from build123d import *

# Parameters (mm, degrees)
F0_R     = 15.24
F0_R_2   = 13.335
F0_R_3   = 8.89
F0_R_4   = 8.382
F1_DEPTH = 5.08
F2_DEPTH = 17.78
F3_DEPTH = 17.78


with BuildPart() as f1:
    # F0 (on Top) → F1 (new body)
    with BuildSketch(Plane.XY):
        Circle(F0_R)
        Circle(F0_R_2, mode=Mode.SUBTRACT)
        Circle(F0_R_2)
        Circle(F0_R_3, mode=Mode.SUBTRACT)
        Circle(F0_R_3)
        Circle(F0_R_4, mode=Mode.SUBTRACT)
        Circle(F0_R_4)
    extrude(amount=F1_DEPTH)

    # F0 (on Top) → F2 (join)
    with BuildSketch(Plane.XY):
        Circle(F0_R)
        Circle(F0_R_2, mode=Mode.SUBTRACT)
    extrude(amount=F2_DEPTH)

    # F0 (on Top) → F3 (join)
    with BuildSketch(Plane.XY):
        Circle(F0_R_3)
        Circle(F0_R_4, mode=Mode.SUBTRACT)
    extrude(amount=F3_DEPTH)


solid = f1.part
Here's how the part is built. I have some questions about the finished solid (model axes, mm). A direction names the side the tool comes from. Round coordinates to 2 decimals unless told otherwise and drop trailing zeros. Write each loop counter-clockwise with the first axis right and the second up, starting at its lowest first coordinate (ties: lowest second). Pieces come first, ordered by that corner, then holes.
1. If we mould it in two halves opening along Y, with no side actions, what happens to faces 3 (the cylindrical face through (-1.93, -8.68, 11.34)), 4 (the flat face through (-3, 8, 17.78)), 5 (the cylindrical face through (-3.3, -14.88, 8.77))? For each: released by +Y, released by -Y, zero draft, split by the parting line, or undercut.
2. Suppose I cut it at A-A (y = 0). List the corners of the cut face in (x, z) for me (3 decimals).
3. For faces 1 (the flat face through (0, 0, 0)), 2 (the cylindrical face through (-1.74, 13.22, 11.34)), which set-ups out of +Z, -Z, +X, -X, +Y, -Y let a thin tool reach every point of the face, with its end or its side?
4. I need wall thicknesses on L1, parallel to Y at x = 0, z = 10.75 (3 decimals); L2, parallel to Y at x = 4.5, z = 10.5; L3, parallel to Z at x = 6.5, y = 0. Which ranges of each line are inside material? Lowest first, please.
5. Suppose I cut it at D-D (z = 2.5). List the corners of the cut face in (x, y) for me, and give its area (3 significant figures).
6. Will these pins go through, and if not, where does the flat tip stop? pin 1 Ø1.5 at (y, z) = (3.5, 12.5) entering from -X; pin 2 Ø5 at (x, y) = (-3, 0) entering from +Z; pin 3 Ø4 at (x, z) = (-9.5, 11) entering from +Y.
7. Suppose I cut it at B-B (z = 9). List the corners of the cut face in (x, y) for me (3 decimals), and give its area (3 significant figures).
Answer sheet:
1. face 3: undercut
1. face 4: zero draft
1. face 5: split by the parting line
2. outline: (-15.24, 0) - (15.24, 0) - (15.24, 17.78) - (13.335, 17.78) - (13.335, 5.08) - (8.89, 5.08) - (8.89, 17.78) - (8.382, 17.78) - (8.382, 5.08) - (-8.382, 5.08) - (-8.382, 17.78) - (-8.89, 17.78) - (-8.89, 5.08) - (-13.335, 5.08) - (-13.335, 17.78) - (-15.24, 17.78) - close
3. face 1: -Z, +X, -X, +Y, -Y
3. face 2: +Z
4. L1: y = -15.24 to -13.335, -8.89 to -8.382, 8.382 to 8.89, 13.335 to 15.24
4. L2: y = -14.56 to -12.55, -7.67 to -7.07, 7.07 to 7.67, 12.55 to 14.56
4. L3: z = 0 to 5.08
5. outline: circle Ø30.48 at (0, 0)
5. area: 730 mm2
6. pin 1: stops at x = -14.99
6. pin 2: stops at z = 5.08
6. pin 3: stops at y = 13.27
7. outline: circle Ø30.48 at (0, 0); circle Ø17.78 at (0, 0); hole circle Ø26.67 at (0, 0); hole circle Ø16.764 at (0, 0)
7. area: 199 mm2
